Geometry: final body of the model. Coordinates: model frame, mm. A direction names the side the tool comes from. Give positions to 0.01 mm unless a question says otherwise; leave off trailing zeros. Loops run counter-clockwise (first coordinate to the right, second up) from the corner with the lowest first, then second, coordinate; pieces in that order, holes last. Notation, with made-up numbers: (41, 72.5) -> (63, 72.5) arc R15 cw to (63, 96.5) -> close; hole circle Ø8 at (-20, -2). An arc over 180 degrees is marked (long way). One line per question, with ' | ' between items. Start each with the question number.
Item 1: Section A-A on y = -3.75. Return loops of the section in (x, z).
Item 2: Mould query, pull axis X, two halves, no side actions, for faces 1 (the flat face through (-106, -3, -114.501)), 2 (the flat face through (-181.531, -3, -98)), 3 (the flat face through (8, -3, -108.151)). Classes: released by +X, released by -X, zero draft, split by the parting line, or undercut.
Item 3: Pin query (flat end, axial travel): P1, Ø1.9, axis at x = 181.5, y = -1.5, coming from the -Z side; P2, Ø3, axis at x = -184.5, y = -4.5, coming from the -Z side; P3, Ø3, axis at x = 202, y = -2.5, coming from the +Z side. Return the tip coordinate at first contact, or that it passes through.
Item 4: Set-up query: faces 4 (the flat face through (-181.531, -3, -54)), 5 (the flat face through (-79.931, -3, -111)), 6 (the flat face through (199.469, -3, -99)), 7 (the flat face through (148.669, -3, -42)). Return all of +Z, -Z, +X, -X, +Y, -Y with unobstructed straight access to the full face (end or side cutting, diameter ignored); none if empty.
Item 5: Section C-C on x = -153.5. Return loops of the section in (y, z), then the cut area to 3 significant figures.
Item 6: Section B-B on z = -59. Return loops of the section in (x, y).
Item 7: Material intervals for line 1 along Z through (x, y) = (-137, -0.5); line 2 along X through (y, z) = (-1, -108), sorted ascending. Write a range as [from, to].
from build123d import *

# Parameters (mm, degrees)
F0_W     = 50.8
F0_H     = 6.35
F0_W_2   = 6.35
F0_H_2   = 25.4
F1_DEPTH = 6.35


with BuildPart() as f1:
    # F0 (on Front) → F1 (new body)
    with BuildSketch(Plane.XZ):
        Polygon((-181.531138, -89.100668), (-181.531138, -108.150668), (-130.731138, -108.150668), (-79.931138, -108.150668), (97.868862, -108.150668), (148.668862, -108.150668), (199.468862, -108.150668), (199.468862, -89.100668), (199.468862, -63.700668), (199.468862, -44.650668), (148.668862, -44.650668), (97.868862, -44.650668), (-79.931138, -44.650668), (-130.731138, -44.650668), (-181.531138, -44.650668), (-181.531138, -63.700668), align=None)
        with Locations((-105.331138, -41.475668)):
            Rectangle(F0_W, F0_H)
        with Locations((-184.706138, -76.400668)):
            Rectangle(F0_W_2, F0_H_2)
        with Locations((-105.331138, -111.325668)):
            Rectangle(F0_W, F0_H)
        with Locations((123.268862, -111.325668)):
            Rectangle(F0_W, F0_H)
        with Locations((123.268862, -41.475668)):
            Rectangle(F0_W, F0_H)
        with Locations((202.643862, -76.400668)):
            Rectangle(F0_W_2, F0_H_2)
    extrude(amount=F1_DEPTH)


solid = f1.part
Result sheet:
1) outline: (-187.88, -89.1) -> (-181.53, -89.1) -> (-181.53, -108.15) -> (-130.73, -108.15) -> (-130.73, -114.5) -> (-79.93, -114.5) -> (-79.93, -108.15) -> (97.87, -108.15) -> (97.87, -114.5) -> (148.67, -114.5) -> (148.67, -108.15) -> (199.47, -108.15) -> (199.47, -89.1) -> (205.82, -89.1) -> (205.82, -63.7) -> (199.47, -63.7) -> (199.47, -44.65) -> (148.67, -44.65) -> (148.67, -38.3) -> (97.87, -38.3) -> (97.87, -44.65) -> (-79.93, -44.65) -> (-79.93, -38.3) -> (-130.73, -38.3) -> (-130.73, -44.65) -> (-181.53, -44.65) -> (-181.53, -63.7) -> (-187.88, -63.7) -> close
2) face 1: zero draft | face 2: released by -X | face 3: undercut
3) P1: stops at z = -108.15 | P2: stops at z = -89.1 | P3: stops at z = -63.7
4) face 4: +Z, -X, +Y, -Y | face 5: -Z, +Y, -Y | face 6: -Z, +X, +Y, -Y | face 7: +Z, +X, +Y, -Y
5) outline: (-6.35, -108.15) -> (0, -108.15) -> (0, -44.65) -> (-6.35, -44.65) -> close | area: 403 mm²
6) outline: (-181.53, -6.35) -> (199.47, -6.35) -> (199.47, 0) -> (-181.53, 0) -> close
7) line 1: z = [-108.15, -44.65] | line 2: x = [-181.53, 199.47]
